from build123d import *

# Parameters (mm, degrees)
F0_W     = 94.170756
F0_H     = 78.479818
F1_DEPTH = 25.4
F2_R     = 17.056969
F3_DEPTH = 25.4
F5_DEPTH = 94.171757


with BuildPart() as f1:
    # F0 (on Top) → F1 (new body)
    with BuildSketch(Plane.XY):
        Rectangle(F0_W, F0_H)
    extrude(amount=F1_DEPTH)

    # F2 (on face) → F3 (join)
    with BuildSketch(Plane.XY.offset(25.4)):
        Circle(F2_R)
    extrude(amount=F3_DEPTH)

    # F4 (on face) → F5 (cut, through all)
    with BuildSketch(Plane.YZ.offset(47.085378)):
        Polygon((17.056969, 50.8), (-17.056969, 50.8), (17.056969, 33.430997), align=None)
    extrude(amount=-F5_DEPTH, mode=Mode.SUBTRACT)


solid = f1.part
Model file for the job. Use its own axes, mm. A direction names the side the tool comes from. Coordinates: 2 decimals unless noted, no trailing zeros. Order: outer loops, then holes, each group sorted by start corner. A loop starts at its lowest first (then second) coordinate and runs counter-clockwise, first axis right, second up. Notation, with made-up numbers: (46, 81.5) -> (65, 81.5) arc R26 cw to (65, 105.5) -> close; hole circle Ø8 at (77.5, 12.5). An arc over 180 degrees is marked (long way). Return JSON: item names as keys, results as strings. Group by question number.
Item 1: Tool access for faces 1 (the cylindrical face through (-3.7, -16.65, 35.1)), 2 (the flat face through (-1, 39.24, 13)): list every direction of +Z, -Z, +X, -X, +Y, -Y with a clear straight run to the whole face (end or side of a thin tool).
Item 2: Saw through at B-B on y = -15. Write the cut outline in (x, z), then the cut area to 3 significant figures.
Item 3: Saw through at C-C on z = 45. Write the cut outline in (x, y), then the cut area to 3 significant figures.
Item 4: Flat gauge pins, fed straight in: P1, Ø5, axis at y = -17, z = 31, coming from the +X side; P2, Ø3, axis at x = -9, z = 43, coming from the +Y side; P3, Ø1, axis at x = 8, y = 25, coming from the +Z side. Where does each tip first touch, or does it go through?
Item 5: Wall check: line 1 along Z through (x, y) = (6.5, -33.5); line 2 along Y through (x, z) = (-2, 45); line 3 along X through (y, z) = (10.5, 30). Give the ranges that are in metal, low to high. Write a range as [from, to].
Item 6: Saw through at D-D on y = 20.5. Write the cut outline in (x, z), then the cut area to 3 significant figures.
Item 7: Saw through at A-A on x = 0. Write the cut outline in (y, z).
Values found:
{
 "1": {"face 1": "+Z", "face 2": "+Z, -Z, +X, -X, +Y"},
 "2": {"outline": "(-47.09, 0) -> (47.09, 0) -> (47.09, 25.4) -> (8.12, 25.4) -> (8.12, 49.75) -> (-8.12, 49.75) -> (-8.12, 25.4) -> (-47.09, 25.4) -> close", "area": "2,790 mm2"},
 "3": {"outline": "(-16.09, -5.67) arc R17.06 ccw to (16.09, -5.67) -> close", "area": "267 mm2"},
 "4": {"P1": "stops at x = 8.98", "P2": "stops at y = 1.21", "P3": "stops at z = 25.4"},
 "5": {"line 1": "z = [0, 25.4]", "line 2": "y = [-16.94, -5.67]", "line 3": "x = [-13.44, 13.44]"},
 "6": {"outline": "(-47.09, 0) -> (47.09, 0) -> (47.09, 25.4) -> (-47.09, 25.4) -> close", "area": "2,390 mm2"},
 "7": {"outline": "(-39.24, 0) -> (39.24, 0) -> (39.24, 25.4) -> (17.06, 25.4) -> (17.06, 33.43) -> (-17.06, 50.8) -> (-17.06, 25.4) -> (-39.24, 25.4) -> close"}
}
